```python
from build123d import *

# Parameters (mm, degrees)
F0_R     = 88.5
F0_R_2   = 76
F1_DEPTH = 160
F2_R     = 88.458341
F3_DEPTH = 31
F4_R     = 12.7
F5_DEPTH = 31


with BuildPart() as f1:
    # F0 (on Top) → F1 (new body)
    with BuildSketch(Plane.XY):
        Circle(F0_R)
        Circle(F0_R_2, mode=Mode.SUBTRACT)
    extrude(amount=F1_DEPTH)

    # F2 (on face) → F3 (join)
    with BuildSketch(Plane(origin=(0, 0, 0), x_dir=(1, 0, 0), z_dir=(0, 0, -1))):
        Circle(F2_R)
    extrude(amount=F3_DEPTH)

    # F4 (on face) → F5 (cut, through all)
    with BuildSketch(Plane(origin=(0, 0, -31), x_dir=(1, 0, 0), z_dir=(0, 0, -1))):
        Circle(F4_R)
    extrude(amount=-F5_DEPTH, mode=Mode.SUBTRACT)


solid = f1.part
```
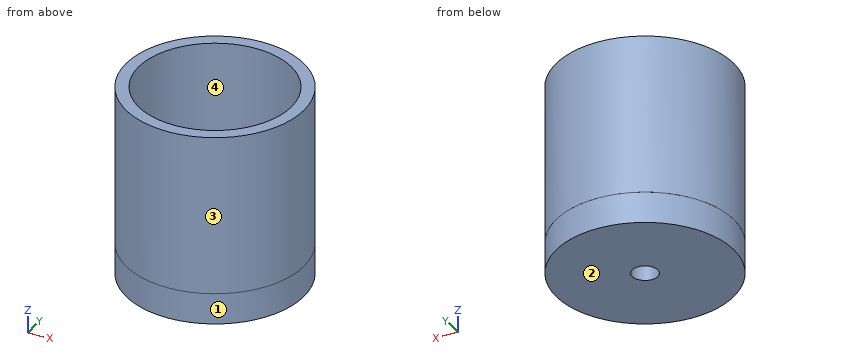
The model under review builds one solid part; all positions refer to its coordinate system, in mm. Face numbers are marked on the shaded views. A direction names the side the tool comes from. Coordinates: 2 decimals unless noted, no trailing zeros. Write each loop counter-clockwise with the first axis right and the second up, starting at its lowest first coordinate (ties: lowest second). Pieces come first, ordered by that corner, then holes. Notation, with made-up numbers: (54.25, 45) - (77.25, 45) arc R23 ccw to (77.25, 61) - close; hole circle Ø9 at (72.25, 11). An arc over 180 degrees is marked (long way). Write item = value, one per line.
(1) For line 1 (X direction, y = 0, z = -16.5); line 2 (Y direction, x = 0, z = 81.5), list the stretches that pass through material, from the lowest coordinate up. Write a range as [from, to].
Result sheet:
line_1 = [-88.46, -12.7], [12.7, 88.46]
line_2 = [-88.5, -76], [76, 88.5]
(2) Mouldability with a two-part tool opening along Z and no side actions: class the marked faces 1 and 2 as pulls with the +Z half, pulls with the -Z half, needs draft (parallel to the pull), parting line crosses it, or undercut.
Result sheet:
face_1 = needs draft
face_2 = pulls with the -Z half
(3) Machinability: for the marked faces 3 and 4, which of the approach directions +Z, -Z, +X, -X, +Y, -Y give a long, thin tool a straight path to every point of the face, cutting with its end or side? Answer none if there is none.
Result sheet:
face_3 = +Z, -Z
face_4 = +Z
(4) Consider section A-A, the plane x = 0. Give the boundary of the cut face in (y, z), then the cut area to 3 significant figures.
Result sheet:
outline = (-88.5, 0) - (-88.46, 0) - (-88.46, -31) - (-12.7, -31) - (-12.7, 0) - (-76, 0) - (-76, 160) - (-88.5, 160) - close; (12.7, -31) - (88.46, -31) - (88.46, 0) - (88.5, 0) - (88.5, 160) - (76, 160) - (76, 0) - (12.7, 0) - close
area = 8,700 mm^2
(5) Consider section D-D, the plane x = -60.5. Give the boundary of the cut face in (y, z), then the cut area to 3 significant figures.
Result sheet:
outline = (-64.59, 0) - (-64.53, 0) - (-64.53, -31) - (64.53, -31) - (64.53, 0) - (64.59, 0) - (64.59, 160) - (46, 160) - (46, 0) - (-46, 0) - (-46, 160) - (-64.59, 160) - close
area = 9,950 mm^2
(6) Consider section C-C, the plane z = 27.5. Give the boundary of the cut face in (x, y).
Result sheet:
outline = circle Ø177 at (0, 0); hole circle Ø152 at (0, 0)
(7) For P1, Ø6, axis at x = -68.5, z = 48.5, coming from the -Y side; P2, Ø4, axis at y = -37.5, z = 55, coming from the +X side; P3, Ø8, axis at x = 62, z = 2, coming from the +Y side, all flat-tipped, find the tip position at first contact; note any pin that passes through.
Result sheet:
P1 = -59.51
P2 = 81.07
P3 = 66.84
